Source: CAD feature listing. Evaluate the final solid. Frame: model axes, mm. A direction names the side the tool comes from. Give positions to 0.01 mm unless a question says otherwise; leave off trailing zeros. Write each loop counter-clockwise with the first axis right and the second up, starting at its lowest first coordinate (ties: lowest second). Pieces come first, ordered by that corner, then holes. Notation, with made-up numbers: M 86,52.5 L 97,52.5 A30 ccw 97,88.5 Z; hole C 52,66.5 d9. An arc over 180 degrees is marked long. Return JSON: item names as keys, results as strings.
```python
from build123d import *

# Parameters (mm, degrees)
F0_R     = 10.4764033566
F1_DEPTH = 128.524
F2_R     = 9.8113639175
F3_R     = 17.037591744
F4_DEPTH = 16.764
F5_R     = 5.08
F6_R     = 5.08
F7_DEPTH = 68.834
F8_R     = 5.08


with BuildPart() as f1:
    # F0 (on Front) → F1 (new body)
    with BuildSketch(Plane.XZ):
        Circle(F0_R)
    extrude(amount=F1_DEPTH)

    # F2
    f2_edges = [f1.edges().sort_by_distance(p)[0] for p in [
        (-10.476403, -128.524, 0),
    ]]
    fillet(f2_edges, radius=F2_R)

    # F3 (on Front) → F4 (join)
    with BuildSketch(Plane.XZ):
        Circle(F3_R)
    extrude(amount=-F4_DEPTH)

    # F5
    f5_edges = [f1.edges().sort_by_distance(p)[0] for p in [
        (-17.037592, 16.764, 0),
    ]]
    fillet(f5_edges, radius=F5_R)

    # F6
    f6_edges = [f1.edges().sort_by_distance(p)[0] for p in [
        (-17.037592, 0, 0),
    ]]
    fillet(f6_edges, radius=F6_R)

    # F7 (add): a face of the model
    f7_faces = [f1.faces().sort_by_distance(p)[0] for p in [
        (0, 16.764, 0),
    ]]
    extrude(f7_faces, amount=F7_DEPTH)

    # F8
    f8_edges = [f1.edges().sort_by_distance(p)[0] for p in [
        (-11.957592, 85.598, 0),
    ]]
    fillet(f8_edges, radius=F8_R)


solid = f1.part
```
1) Cut plane A-A, the plane y = -101. Return the cut outline in (x, z), then the cut area to 3 significant figures.
Numbers:
{"outline": "C 0,0 d20.95", "area": "345 mm²"}
2) Set-up query: faces 1 (the face through (16.25, 8.34, 5.12)), 2 (the face through (0, 0, -11)), 3 (the face through (-8.813, 48.195, 8.082)). Return all of +Z, -Z, +X, -X, +Y, -Y with unobstructed straight access to the full face (end or side cutting, diameter ignored); none if empty.
Numbers:
{"face 1": "+Y, -Y", "face 2": "-Y", "face 3": "+Y"}
3) Line query: line 1 (Y direction, x = -11.5, z = -4.5); line 2 (Y direction, x = 9.5, z = 13); line 3 (Z direction, x = -1, y = -39). Output: solid intervals per line, ascending. Write a range as [from, to].
Numbers:
{"line 1": "y = [0.02, 16.75]", "line 2": "y = [2.14, 14.62]", "line 3": "z = [-10.43, 10.43]"}
4) Cut plane B-B, the plane y = 66. Return the cut outline in (x, z).
Numbers:
{"outline": "C 0,0 d23.92"}
5) Contact query for flat-ended pins moving along their axis: pin 1 Ø8 at (x, y) = (7.5, -47.5) entering from +Z; pin 2 Ø5 at (y, z) = (-35, 7.5) entering from +X; pin 3 Ø4 at (y, z) = (-20, -3.5) entering from -X. Output: stop coordinate, or through.
Numbers:
{"pin 1": "stops at z = 9.87", "pin 2": "stops at x = 9.21", "pin 3": "stops at x = -10.37"}
